Can you work these out from the model? Positions are in its coordinate system, mm. Face numbers are marked on the shaded views. A direction names the side the tool comes from. Coordinates: 2 decimals unless noted, no trailing zeros. Order: outer loops, then holes, each group sorted by start corner. A loop starts at its lowest first (then second) coordinate and runs counter-clockwise, first axis right, second up. Notation, with made-up numbers: (-1.75, 27) -> (16.25, 27) arc R33 cw to (16.25, 59) -> close; hole circle Ø10 at (28.5, 39). An arc over 180 degrees is marked (long way). Return JSON: item names as keys, results as strings. Group by question number.
1) If we section it at A-A, the plane z = 12: Please give me the cut outline in (x, y).
2) Thinking about a two-plate mould opening in X: for the marked faces 3, 4, 5 and 6, which applies, +X half, -X half, draft (parallel to the pull), parting line (faces both ways), or undercut?
3) For pin 1 (1.6 mm diameter, centred on x = 23, z = 12.5, fed in from -Y); pin 2 (15 mm diameter, centred on x = 15.5, y = 37, fed in from -Z); pin 3 (0.6 mm diameter, centred on x = 28.5, z = 15.5, fed in from +Y); pin 4 (4 mm diameter, centred on x = 38, z = -12.5, fed in from -Y), each with a flat end and sliding along its axis, tell me the tip position at first contact or that it passes through.
4) For the marked faces 1 and 2, which set-ups out of +Z, -Z, +X, -X, +Y, -Y let a thin tool reach every point of the face, with its end or its side?
5) If we section it at B-B, the plane y = 20: Please give me the cut outline in (x, z), then the cut area to 3 significant figures.
6) If we section it at C-C, the plane z = -25: Please give me the cut outline in (x, y), then the cut area to 3 significant figures.
7) If we section it at D-D, the plane y = 28.5: Please give me the cut outline in (x, z), then the cut area to 3 significant figures.
8) If I drill on probe 1 along X at (y, z) = (32, -34); probe 2 along X at (y, z) = (29, 10); probe 3 along Y at (x, z) = (23, 12), over which ranges is the centre line in solid material (lowest first)? Write a range as from..to.
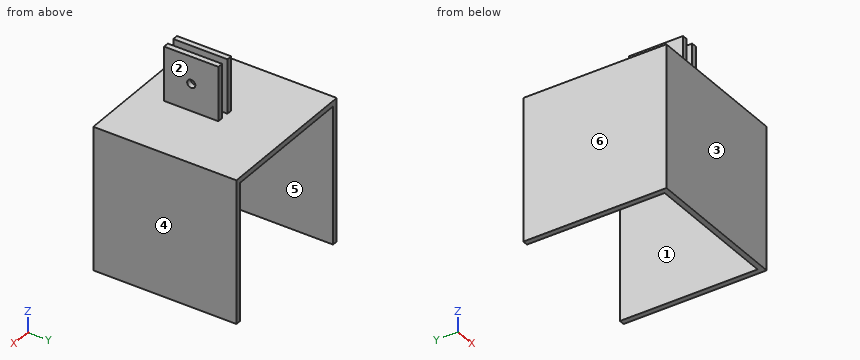
from build123d import *

# Parameters (mm, degrees)
SKETCH1_W                = 50.8
SKETCH1_H                = 50.8
BOSS_EXTRUDE1_DEPTH      = 2
BOSS_EXTRUDE2_START      = 2
BOSS_EXTRUDE2_DEPTH      = 50.8
BOSS_EXTRUDE3_DEPTH      = 10
BOSS_EXTRUDE3_DEPTH_BACK = 10
BOSS_EXTRUDE3_START      = 20
SKETCH1_4_W              = 2
SKETCH1_4_H              = 20
CUT_EXTRUDE1_REACH       = 81.519
SKETCH3_R                = 1.5


with BuildPart() as part:
    # Sketch1 → Boss-Extrude1 (new body)
    with BuildSketch(Plane(origin=(0, 0, 0), x_dir=(1, 0, 0), z_dir=(0, 1, 0))):
        Polygon((52.8, -2), (52.8, 50.8), (50.8, 50.8), (50.8, 0), (0, 0), (0, 50.8), (-2, 50.8), (-2, -2), align=None)
        with Locations((25.4, 25.4)):
            Rectangle(SKETCH1_W, SKETCH1_H)
    extrude(amount=BOSS_EXTRUDE1_DEPTH)

    # Sketch1<3> → Boss-Extrude2 (add)
    with BuildSketch(Plane(origin=(0, 0, 0), x_dir=(1, 0, 0), z_dir=(0, 1, 0)).offset(BOSS_EXTRUDE2_START)):
        Polygon((52.8, -2), (52.8, 50.8), (50.8, 50.8), (50.8, 0), (0, 0), (0, 50.8), (-2, 50.8), (-2, -2), align=None)
    extrude(amount=BOSS_EXTRUDE2_DEPTH)

    # Sketch1<4> → Boss-Extrude3 (add, two sides: drawn at the far end of the back side and taken through both)
    with BuildSketch(Plane(origin=(0, 0, 0), x_dir=(1, 0, 0), z_dir=(0, 1, 0)).offset(BOSS_EXTRUDE3_START - BOSS_EXTRUDE3_DEPTH_BACK)):
        with Locations((27.9, -12)):
            Rectangle(SKETCH1_4_W, SKETCH1_4_H)
        with Locations((22.9, -12)):
            Rectangle(SKETCH1_4_W, SKETCH1_4_H)
    extrude(amount=BOSS_EXTRUDE3_DEPTH + BOSS_EXTRUDE3_DEPTH_BACK)

    # Cut-Extrude1: up to this face of the body (flat: up to its plane)
    cut_extrude1_end = Plane(part.part.faces().sort_by_distance((21.9, 20, 12))[0])
    # Sketch3 → Cut-Extrude1 (cut, up to the picked face)
    with BuildSketch(Plane(origin=(28.9, 0, 0), x_dir=(0, 0, -1), z_dir=(1, 0, 0)), mode=Mode.PRIVATE) as cut_extrude1_sk1:
        with Locations((-12, 20)):
            Circle(SKETCH3_R)
    cut_extrude1_tool1 = split(extrude(cut_extrude1_sk1.sketch, amount=-CUT_EXTRUDE1_REACH, mode=Mode.PRIVATE), bisect_by=cut_extrude1_end, keep=Keep.BOTH, mode=Mode.PRIVATE)
    add(cut_extrude1_tool1.solids().sort_by(Axis((28.9, 20, 12), (-1, 0, 0)))[0], mode=Mode.SUBTRACT)


solid = part.part
Result sheet:
{
 "1": {"outline": "(21.9, 10) -> (23.9, 10) -> (23.9, 18.5) -> (21.9, 18.5) -> close; (21.9, 21.5) -> (23.9, 21.5) -> (23.9, 30) -> (21.9, 30) -> close; (26.9, 10) -> (28.9, 10) -> (28.9, 18.5) -> (26.9, 18.5) -> close; (26.9, 21.5) -> (28.9, 21.5) -> (28.9, 30) -> (26.9, 30) -> close"},
 "2": {"face 3": "draft", "face 4": "+X half", "face 5": "undercut", "face 6": "-X half"},
 "3": {"pin 1": "stops at y = 10", "pin 2": "stops at z = 0", "pin 3": "stops at y = 30", "pin 4": "stops at y = 0"},
 "4": {"face 1": "-Z, +Y", "face 2": "+Z, +X, +Y, -Y"},
 "5": {"outline": "(-2, -50.8) -> (0, -50.8) -> (0, 0) -> (50.8, 0) -> (50.8, -50.8) -> (52.8, -50.8) -> (52.8, 2) -> (28.9, 2) -> (28.9, 10.5) -> (26.9, 10.5) -> (26.9, 2) -> (23.9, 2) -> (23.9, 10.5) -> (21.9, 10.5) -> (21.9, 2) -> (-2, 2) -> close; (21.9, 13.5) -> (23.9, 13.5) -> (23.9, 22) -> (21.9, 22) -> close; (26.9, 13.5) -> (28.9, 13.5) -> (28.9, 22) -> (26.9, 22) -> close", "area": "381 mm2"},
 "6": {"outline": "(-2, 0) -> (52.8, 0) -> (52.8, 52.8) -> (50.8, 52.8) -> (50.8, 2) -> (0, 2) -> (0, 52.8) -> (-2, 52.8) -> close", "area": "313 mm2"},
 "7": {"outline": "(-2, -50.8) -> (0, -50.8) -> (0, 0) -> (50.8, 0) -> (50.8, -50.8) -> (52.8, -50.8) -> (52.8, 2) -> (28.9, 2) -> (28.9, 22) -> (26.9, 22) -> (26.9, 2) -> (23.9, 2) -> (23.9, 22) -> (21.9, 22) -> (21.9, 2) -> (-2, 2) -> close", "area": "393 mm2"},
 "8": {"probe 1": "x = -2..0, 50.8..52.8", "probe 2": "x = 21.9..23.9, 26.9..28.9", "probe 3": "y = 10..18.5, 21.5..30"}
}
